Verification items for the finished model (mm, model axes). Face numbers are marked on the shaded views. A direction names the side the tool comes from. Round coordinates to 2 decimals unless told otherwise and drop trailing zeros. Write each loop counter-clockwise with the first axis right and the second up, starting at its lowest first coordinate (ties: lowest second). Pieces come first, ordered by that corner, then holes. Notation, with made-up numbers: (81, 61.25) -> (90, 61.25) arc R18 ccw to (90, 66.25) -> close; hole circle Ø5 at (7.25, -5). An arc over 180 degrees is marked (long way). Answer as a JSON object with one key per item and string values. Group by question number.
(1) Sectioned sample at C-C on x = 0. Record the cut outline in (y, z), and give its area (3 significant figures).
(2) Set-up check for the marked faces 5, 6, 7, 8 and 9: record each of +Z, -Z, +X, -X, +Y, -Y from which the full face is reachable in a straight line by a thin tool's end or side.
(3) Sectioned sample at D-D on z = 140.5. Record the cut outline in (x, y).
(4) Sectioned sample at B-B on y = -42. Record the cut outline in (x, z), and give its area (3 significant figures).
(5) Sectioned sample at A-A on x = -56. Record the cut outline in (y, z).
(6) Scan lines: L1, parallel to X at y = -98, z = -11; L2, parallel to Y at x = -25, z = 136.5; L3, parallel to Z at x = -27, y = -76. Record each from-to range of solid material in increasing order. Write a range as from..to.
(7) Gauge pin test, flat ends, axial feed: pin 1 Ø6 at (x, z) = (-27.5, 106.5) entering from +Y; pin 2 Ø8 at (y, z) = (-48.5, 90.5) entering from +X; pin 3 Ø4 at (y, z) = (-47.5, 123.5) entering from -X; pin 4 Ø8 at (y, z) = (-34, 132.5) entering from +X. Record the tip position at first contact, or that the pin passes through.
(8) Draft check along Y on the marked faces 1, 2, 3 and 4. Enter one of: released by +Y, released by -Y, zero draft, split by the parting line, or undercut.
```python
from build123d import *

# Parameters (mm, degrees)
SKETCH_2_R      = 25.25
EXTRUDE_1_DEPTH = 3
SKETCH_3_R      = 11.5
EXTRUDE_2_DEPTH = 77
SKETCH_4_R      = 11.5
EXTRUDE_3_DEPTH = 72
SKETCH_5_R      = 25.25
EXTRUDE_4_DEPTH = 3
EXTRUDE_START   = 3
SKETCH_6_R      = 25.25
EXTRUDE_5_DEPTH = 3
FILLET_1_R      = 10
SKETCH_7_R      = 11.5
EXTRUDE_6_DEPTH = 53
SKETCH_8_W      = 145
SKETCH_8_H      = 100
EXTRUDE_7_DEPTH = 41


with BuildPart() as part:
    # Sketch 2 → Extrude 1 (new body)
    with BuildSketch(Plane(origin=(0, 0, 0), x_dir=(1, 0, 0), z_dir=(0, 1, 0))):
        with Locations(Location((0, 0, 0), (0, 0, 270))):
            Circle(SKETCH_2_R)
    extrude(amount=-EXTRUDE_1_DEPTH)

    # Sketch 3 → Extrude 2 (add)
    with BuildSketch(Plane.XZ.offset(3)):
        with Locations(Location((0, 0, 0), (0, 0, 270))):
            Circle(SKETCH_3_R)
    extrude(amount=EXTRUDE_2_DEPTH)

    # Sketch 4 → Extrude 3 (add, symmetric)
    with BuildSketch(Plane(origin=(0, 0, 0), x_dir=(0, 0, -1), z_dir=(1, 0, 0))):
        with Locations((0, -80)):
            Circle(SKETCH_4_R)
    extrude(amount=EXTRUDE_3_DEPTH, both=True)

    # Sketch 5 → Extrude 4 (add)
    with BuildSketch(Plane(origin=(72, 0, 0), x_dir=(0, 0, -1), z_dir=(1, 0, 0))):
        with Locations((0, -80)):
            Circle(SKETCH_5_R)
    extrude(amount=EXTRUDE_4_DEPTH)

    # Sketch 6 → Extrude 5 (add)
    with BuildSketch(Plane.ZY.offset(72).offset(EXTRUDE_START)):
        with Locations(Location((0, -80, 0), (0, 0, 180))):
            Circle(SKETCH_6_R)
    extrude(amount=-EXTRUDE_5_DEPTH)

    # Fillet 1
    fillet_1_edges = [part.edges().sort_by_distance(p)[0] for p in [
        (72, -80, 11.5),
        (-72, -80, 11.5),
        (0, -3, 11.5),
    ]]
    fillet(fillet_1_edges, radius=FILLET_1_R)

    # Sketch 7 → Extrude 6 (add)
    with BuildSketch(Plane.XY):
        with Locations((0, -80)):
            Circle(SKETCH_7_R)
    extrude(amount=EXTRUDE_6_DEPTH)

    # Sketch 8 → Extrude 7 (add, symmetric)
    with BuildSketch(Plane(origin=(0, -80, 0), x_dir=(1, 0, 0), z_dir=(0, 1, 0))):
        with Locations((0, -103)):
            Rectangle(SKETCH_8_W, SKETCH_8_H)
    extrude(amount=EXTRUDE_7_DEPTH, both=True)


solid = part.part
```
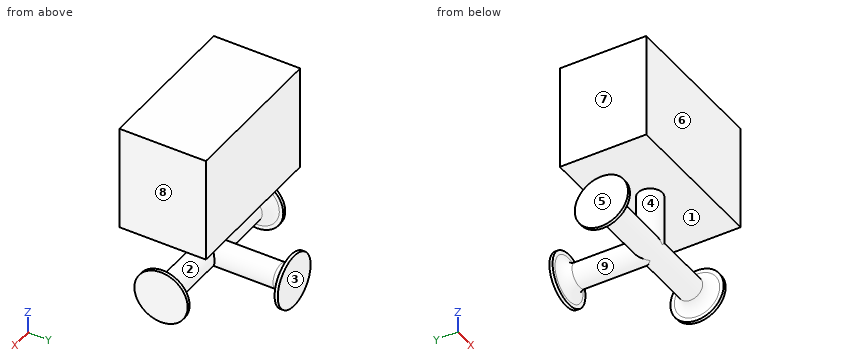
Computed values:
{
 "1": {"outline": "(-121, 53) -> (-91.5, 53) -> (-91.5, 0) arc R11.5 ccw to (-80, -11.5) -> (-13, -11.5) arc R10 cw to (-3, -21.5) -> (-3, -25.25) -> (0, -25.25) -> (0, 25.25) -> (-3, 25.25) -> (-3, 21.5) arc R10 cw to (-13, 11.5) -> (-68.5, 11.5) -> (-68.5, 53) -> (-39, 53) -> (-39, 153) -> (-121, 153) -> close", "area": "11,400 mm2"},
 "2": {"face 5": "+Z, -Z, -X, +Y, -Y", "face 6": "+Z, -Z, +X, -X, -Y", "face 7": "+Z, -X, +Y, -Y", "face 8": "+Z, +X, +Y, -Y", "face 9": "none"},
 "3": {"outline": "(-72.5, -121) -> (72.5, -121) -> (72.5, -39) -> (-72.5, -39) -> close"},
 "4": {"outline": "(-72.5, 53) -> (72.5, 53) -> (72.5, 153) -> (-72.5, 153) -> close; circle Ø23 at (0, 0)", "area": "14,900 mm2"},
 "5": {"outline": "(-121, 53) -> (-39, 53) -> (-39, 153) -> (-121, 153) -> close; circle Ø23 at (-80, 0)"},
 "6": {"L1": "-75..-71.99, 71.99..75", "L2": "-121..-39", "L3": "-10.78..10.78, 53..153"},
 "7": {"pin 1": "y = -39", "pin 2": "x = 72.5", "pin 3": "x = -72.5", "pin 4": "through"},
 "8": {"face 1": "zero draft", "face 2": "undercut", "face 3": "released by +Y", "face 4": "undercut"}
}
